```python
from build123d import *

# Parameters (mm, degrees)
ESQUISSE1_W             = 57
ESQUISSE1_H             = 20.9
ESQUISSE1_R             = 2.25
ESQUISSE1_W_2           = 5.5
ESQUISSE1_H_2           = 10
BOSS_EXTRU_2_DEPTH      = 4
ESQUISSE2_W             = 16.5
ESQUISSE2_H             = 5.5
ESQUISSE2_R             = 2.25
BOSS_EXTRU_3_DEPTH      = 6
ENL_V_START             = -7.5
ESQUISSE4_R             = 2.25
ENL_V_MAT_EXTRU_2_DEPTH = 5.5


with BuildPart() as part:
    # Esquisse1 → Boss.-Extru.2 (new body)
    with BuildSketch(Plane.XY):
        with Locations((28.5, -10.45)):
            Rectangle(ESQUISSE1_W, ESQUISSE1_H)
        with Locations((5, -9)):
            Circle(ESQUISSE1_R, mode=Mode.SUBTRACT)
        with Locations((52, -9)):
            Circle(ESQUISSE1_R, mode=Mode.SUBTRACT)
        with Locations((34.75, -9)):
            Rectangle(ESQUISSE1_W_2, ESQUISSE1_H_2, mode=Mode.SUBTRACT)
        with Locations((22.25, -9)):
            Rectangle(ESQUISSE1_W_2, ESQUISSE1_H_2, mode=Mode.SUBTRACT)
    extrude(amount=BOSS_EXTRU_2_DEPTH)

    # Esquisse2 → Boss.-Extru.3 (add)
    # profile 1 of 2: a face of its own
    with BuildSketch(Plane.XY.offset(4)):
        with Locations((36.75, -18.15)):
            Rectangle(ESQUISSE2_W, ESQUISSE2_H)
    # profile 2 of 2: a face of its own
    with BuildSketch(Plane.XY.offset(4)):
        Polygon((57, -20.9), (57, 0), (45, 0), (45, -15.4), (45, -20.9), align=None)
        with Locations((52, -9)):
            Circle(ESQUISSE2_R, mode=Mode.SUBTRACT)
    boss_extru_3 = extrude(amount=BOSS_EXTRU_3_DEPTH)

    # Esquisse4 → Enlèv. mat.-Extru.2 (cut)
    # profile 1 of 2: a face of its own
    with BuildSketch(Plane.XY.offset(10).offset(ENL_V_START)):
        Polygon((56.214656965, -9), (54.107328483, -5.35), (49.892671517, -5.35), (47.785343035, -9), (49.892671517, -12.65), (54.107328483, -12.65), align=None)
        with Locations((52, -9)):
            Circle(ESQUISSE4_R, mode=Mode.SUBTRACT)
    # profile 2 of 2: a face of its own
    with BuildSketch(Plane.XY.offset(10).offset(ENL_V_START)):
        Polygon((57, -5.35), (54.107328483, -5.35), (56.214656965, -9), (54.107328483, -12.65), (57, -12.65), align=None)
    enl_v_mat_extru_2 = extrude(amount=ENL_V_MAT_EXTRU_2_DEPTH, mode=Mode.SUBTRACT)

    # Symétrie3: Boss.-Extru.3, Enlèv. mat.-Extru.2 across plane
    add(boss_extru_3.mirror(Plane(origin=(28.5, 0, 0), x_dir=(0, 0, 1), z_dir=(1, 0, 0))))
    add(enl_v_mat_extru_2.mirror(Plane(origin=(28.5, 0, 0), x_dir=(0, 0, 1), z_dir=(1, 0, 0))), mode=Mode.SUBTRACT)


solid = part.part
```
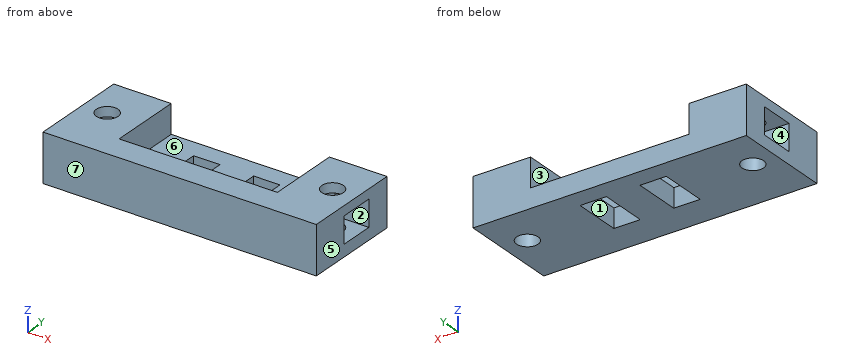
Read the model definition and answer for the solid it produces. Units are mm, in the model's axes. Face numbers are marked on the shaded views. A direction names the side the tool comes from. Round coordinates to 2 decimals unless told otherwise and drop trailing zeros. Write each loop counter-clockwise with the first axis right and the second up, starting at its lowest first coordinate (ties: lowest second). Pieces come first, ordered by that corner, then holes. Notation, with made-up numbers: (-31.75, 48) -> (22.25, 48) arc R16 ccw to (22.25, 58) -> close; hole circle Ø8 at (22.5, 0). An arc over 180 degrees is marked (long way). Answer in a Markdown table with one row per item. Add a question column.
1) Find section C-C, the plane z = 1. Determine the outline of the cut face in (x, y).
2) Determine the mould class of the marked faces 5, 6 and 7 for opening direction X: pulls with the +X half, pulls with the -X half, needs draft (parallel to the pull), parting line crosses it, or undercut.
3) Which of the six approach directions +Z, -Z, +X, -X, +Y, -Y give full straight-line access (tool end or side, diameter ignored) to the marked faces 1, 2, 3 and 4?
4) Find section D-D, the plane x = 5. Determine the outline of the cut face in (y, z), and give its area (3 significant figures).
5) Given P1, Ø1.8, axis at x = 20.5, z = 6.5, coming from the +Y side; P2, Ø3.5, axis at x = 52, y = -9, coming from the +Z side, each flat-ended and moving along its own axis, determine where each tip first touches the part or whether it passes through.
6) Consider line 1 (Z direction, x = 6.5, y = -5.5); line 2 (Y direction, x = 52, z = 1.5); line 3 (X direction, y = -4, z = 7). Determine where each line is inside the solid, lowest interval first.
7) Find section B-B, the plane z = 9. Determine the outline of the cut face in (x, y).
8) Find section A-A, the plane x = 20. Determine the outline of the cut face in (y, z), and give its area (3 significant figures).
Findings below:
| question | item | result |
|---|---|---|
| 1 | outline | (0, -20.9) -> (57, -20.9) -> (57, 0) -> (0, 0) -> close; hole circle Ø4.5 at (5, -9); hole (19.5, -14) -> (25, -14) -> (25, -4) -> (19.5, -4) -> close; hole (32, -14) -> (37.5, -14) -> (37.5, -4) -> (32, -4) -> close; hole circle Ø4.5 at (52, -9) |
| 2 | face 5 | pulls with the +X half |
| 2 | face 6 | undercut |
| 2 | face 7 | needs draft |
| 3 | face 1 | +Z, -Z |
| 3 | face 2 | +X |
| 3 | face 3 | +Z, +Y |
| 3 | face 4 | -X |
| 4 | outline | (-20.9, 0) -> (-11.25, 0) -> (-11.25, 2.5) -> (-12.65, 2.5) -> (-12.65, 8) -> (-11.25, 8) -> (-11.25, 10) -> (-20.9, 10) -> close; (-6.75, 0) -> (0, 0) -> (0, 10) -> (-6.75, 10) -> (-6.75, 8) -> (-5.35, 8) -> (-5.35, 2.5) -> (-6.75, 2.5) -> close |
| 4 | area | 149 mm² |
| 5 | P1 | y = -15.4 |
| 5 | P2 | through |
| 6 | line 1 | 0 to 2.5, 8 to 10 |
| 6 | line 2 | -20.9 to -11.25, -6.75 to 0 |
| 6 | line 3 | 0 to 12, 45 to 57 |
| 7 | outline | (0, -20.9) -> (57, -20.9) -> (57, 0) -> (45, 0) -> (45, -15.4) -> (12, -15.4) -> (12, 0) -> (0, 0) -> close; hole circle Ø4.5 at (5, -9); hole circle Ø4.5 at (52, -9) |
| 8 | outline | (-20.9, 0) -> (-14, 0) -> (-14, 4) -> (-15.4, 4) -> (-15.4, 10) -> (-20.9, 10) -> close; (-4, 0) -> (0, 0) -> (0, 4) -> (-4, 4) -> close |
| 8 | area | 76.6 mm² |
